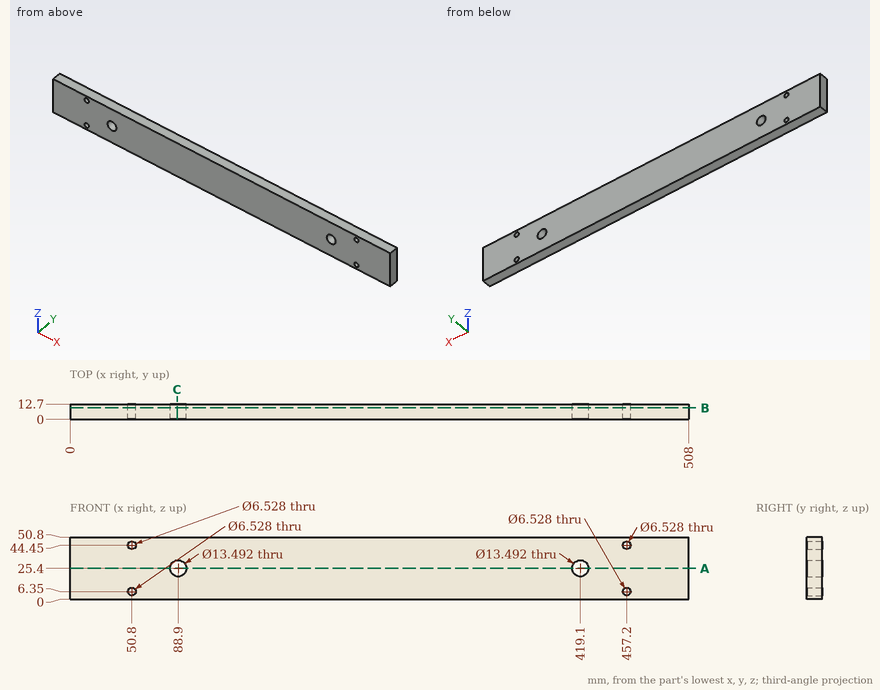
Geometry: see drawing. Coordinates: mm, zero at the bounding-box minimum. Coordinates: 2 decimals unless noted, no trailing zeros. Loops run counter-clockwise (first coordinate to the right, second up) from the corner with the lowest first, then second, coordinate; pieces in that order, holes last.
Q1. Cut plane C-C (x = 88). Output: boundary loops of the cut face in (y, z) (1 decimal).
Q2. Material intervals for line 1 (Z direction, x = 457.2, y = 7.5); line 2 (X direction, y = 1.25, z = 29.5) (1 decimal); line 3 (X direction, y = 4, z = 4) (1 decimal), sorted ascending.
Q3. Cut plane A-A (z = 25.4). Output: boundary loops of the cut face in (x, y).
Q4. Cut plane B-B (y = 9.5). Output: boundary loops of the cut face in (x, z), then the cut area to 3 significant figures.
Working result:
1. outline: (0, 0) - (12.7, 0) - (12.7, 18.7) - (0, 18.7) - close; (0, 32.1) - (12.7, 32.1) - (12.7, 50.8) - (0, 50.8) - close
2. line 1: z = 0 to 3.09, 9.61 to 41.19, 47.71 to 50.8
2. line 2: x = 0 to 83.5, 94.3 to 413.7, 424.5 to 508
2. line 3: x = 0 to 48.5, 53.1 to 454.9, 459.5 to 508
3. outline: (0, 0) - (82.15, 0) - (82.15, 12.7) - (0, 12.7) - close; (95.65, 0) - (412.35, 0) - (412.35, 12.7) - (95.65, 12.7) - close; (425.85, 0) - (508, 0) - (508, 12.7) - (425.85, 12.7) - close
4. outline: (0, 0) - (508, 0) - (508, 50.8) - (0, 50.8) - close; hole circle Ø6.53 at (50.8, 6.35); hole circle Ø6.53 at (50.8, 44.45); hole circle Ø13.49 at (88.9, 25.4); hole circle Ø13.49 at (419.1, 25.4); hole circle Ø6.53 at (457.2, 6.35); hole circle Ø6.53 at (457.2, 44.45)
4. area: 25,400 mm2
